Design review of the part built by this model. Coordinates are the model's own, in mm. Face numbers are marked on the shaded views. A direction names the side the tool comes from. Coordinates: 2 decimals unless noted, no trailing zeros. Loops run counter-clockwise (first coordinate to the right, second up) from the corner with the lowest first, then second, coordinate; pieces in that order, holes last. Notation, with made-up numbers: M 76,4 L 100,4 A8 cw 100,10 Z; hole C -10.75,37 d11. An arc over 180 degrees is marked long. Put each result on its own line as item: value. Start each with the question number.
(1) Take a section at B-B, the plane y = -11. Give the boundary of the cut face in (x, z).
(2) Clearance check with flat-ended pins moving along their axes: pin 1 (10 mm diameter, centred on x = -6, y = 5.5, fed in from -Z); pin 2 (2 mm diameter, centred on y = -0.5, z = -5.5, fed in from -X); pin 3 (2 mm diameter, centred on y = -11.5, z = -1.5, fed in from -X). State where each tip first meets the part, or that it passes through.
(3) Take a section at C-C, the plane z = -9.5. Give the boundary of the cut face in (x, y).
(4) Take a section at D-D, the plane y = 0. Give the boundary of the cut face in (x, z), then the cut area to 3 significant figures.
(5) The part is to be moulded in two halves that separate along Y. For the marked faces 3, 4 and 5, say which applies: +Y half, -Y half, draft (parallel to the pull), parting line (faces both ways), or undercut.
(6) Take a section at A-A, the plane x = 0. Give the boundary of the cut face in (y, z).
(7) For the marked faces 1 and 2, list the 3-axis set-ups (+Z, -Z, +X, -X, +Y, -Y) from which the entire face can be reached by the end or side of a thin tool; tool diameter is ignored.
(8) For probe 1 along Y at (x, z) = (0, 0.7); probe 2 along Y at (x, z) = (-12, -7.5); probe 3 along Z at (x, y) = (4, 8.5), list the stretches that pass through material, from the lowest coordinate up. Write a range as [from, to].
```python
from build123d import *

# Parameters (mm, degrees)
F0_W     = 40
F0_H     = 32
F0_R     = 6.25
F1_DEPTH = 2
F3_START = 13
F3_DEPTH = 3
F4_START = -13
F4_DEPTH = 3
F5_DEPTH = 16


with BuildPart() as f1:
    # F0 (on Top) → F1 (new body)
    with BuildSketch(Plane.XY):
        Rectangle(F0_W, F0_H)
        Circle(F0_R, mode=Mode.SUBTRACT)
    extrude(amount=F1_DEPTH)

    # F2 (on Front) → F3 (join)
    with BuildSketch(Plane.XZ.offset(F3_START)):
        with BuildLine():
            ThreePointArc((18.1261557407, -8.4523652348), (19.5259201424, -4.3287922788), (20, 0))
            Line((20, 0), (18.5, 0))
            ThreePointArc((18.5, 0), (18.0614761317, -4.0041328579), (16.7666940602, -7.8184378422))
            Line((16.7666940602, -7.8184378422), (18.1261557407, -8.4523652348))
        make_face()
        with BuildLine():
            Line((-18.5, 0), (-20, 0))
            ThreePointArc((-20, 0), (-19.5259201424, -4.3287922788), (-18.1261557407, -8.4523652348))
            Line((-18.1261557407, -8.4523652348), (-16.7666940602, -7.8184378422))
            ThreePointArc((-16.7666940602, -7.8184378422), (-18.0614761317, -4.0041328579), (-18.5, 0))
        make_face()
        with BuildLine():
            ThreePointArc((-18.1261557407, -8.4523652348), (0, -20), (18.1261557407, -8.4523652348))
            Line((18.1261557407, -8.4523652348), (16.7666940602, -7.8184378422))
            ThreePointArc((16.7666940602, -7.8184378422), (0, -18.5), (-16.7666940602, -7.8184378422))
            Line((-16.7666940602, -7.8184378422), (-18.1261557407, -8.4523652348))
        make_face()
        with BuildLine():
            ThreePointArc((16.7666940602, -7.8184378422), (18.0614761317, -4.0041328579), (18.5, 0))
            Line((18.5, 0), (0, 0))
            Line((0, 0), (16.7666940602, -7.8184378422))
        make_face()
        with BuildLine():
            Line((0, 0), (-18.5, 0))
            ThreePointArc((-18.5, 0), (-18.0614761317, -4.0041328579), (-16.7666940602, -7.8184378422))
            Line((-16.7666940602, -7.8184378422), (0, 0))
        make_face()
        with BuildLine():
            ThreePointArc((-16.7666940602, -7.8184378422), (0, -18.5), (16.7666940602, -7.8184378422))
            Line((16.7666940602, -7.8184378422), (0, 0))
            Line((0, 0), (-16.7666940602, -7.8184378422))
        make_face()
    extrude(amount=F3_DEPTH)

    # F2 (on Front) → F4 (join)
    with BuildSketch(Plane.XZ.offset(F4_START)):
        with BuildLine():
            ThreePointArc((18.1261557407, -8.4523652348), (19.5259201424, -4.3287922788), (20, 0))
            Line((20, 0), (18.5, 0))
            ThreePointArc((18.5, 0), (18.0614761317, -4.0041328579), (16.7666940602, -7.8184378422))
            Line((16.7666940602, -7.8184378422), (18.1261557407, -8.4523652348))
        make_face()
        with BuildLine():
            Line((-18.5, 0), (-20, 0))
            ThreePointArc((-20, 0), (-19.5259201424, -4.3287922788), (-18.1261557407, -8.4523652348))
            Line((-18.1261557407, -8.4523652348), (-16.7666940602, -7.8184378422))
            ThreePointArc((-16.7666940602, -7.8184378422), (-18.0614761317, -4.0041328579), (-18.5, 0))
        make_face()
        with BuildLine():
            ThreePointArc((-18.1261557407, -8.4523652348), (0, -20), (18.1261557407, -8.4523652348))
            Line((18.1261557407, -8.4523652348), (16.7666940602, -7.8184378422))
            ThreePointArc((16.7666940602, -7.8184378422), (0, -18.5), (-16.7666940602, -7.8184378422))
            Line((-16.7666940602, -7.8184378422), (-18.1261557407, -8.4523652348))
        make_face()
        with BuildLine():
            ThreePointArc((16.7666940602, -7.8184378422), (18.0614761317, -4.0041328579), (18.5, 0))
            Line((18.5, 0), (0, 0))
            Line((0, 0), (16.7666940602, -7.8184378422))
        make_face()
        with BuildLine():
            Line((0, 0), (-18.5, 0))
            ThreePointArc((-18.5, 0), (-18.0614761317, -4.0041328579), (-16.7666940602, -7.8184378422))
            Line((-16.7666940602, -7.8184378422), (0, 0))
        make_face()
        with BuildLine():
            ThreePointArc((-16.7666940602, -7.8184378422), (0, -18.5), (16.7666940602, -7.8184378422))
            Line((16.7666940602, -7.8184378422), (0, 0))
            Line((0, 0), (-16.7666940602, -7.8184378422))
        make_face()
    extrude(amount=-F4_DEPTH)

    # F2 (on Front) → F5 (join, symmetric)
    with BuildSketch(Plane.XZ):
        with BuildLine():
            ThreePointArc((18.1261557407, -8.4523652348), (19.5259201424, -4.3287922788), (20, 0))
            Line((20, 0), (18.5, 0))
            ThreePointArc((18.5, 0), (18.0614761317, -4.0041328579), (16.7666940602, -7.8184378422))
            Line((16.7666940602, -7.8184378422), (18.1261557407, -8.4523652348))
        make_face()
        with BuildLine():
            Line((-18.5, 0), (-20, 0))
            ThreePointArc((-20, 0), (-19.5259201424, -4.3287922788), (-18.1261557407, -8.4523652348))
            Line((-18.1261557407, -8.4523652348), (-16.7666940602, -7.8184378422))
            ThreePointArc((-16.7666940602, -7.8184378422), (-18.0614761317, -4.0041328579), (-18.5, 0))
        make_face()
    extrude(amount=F5_DEPTH, both=True)


solid = f1.part
```
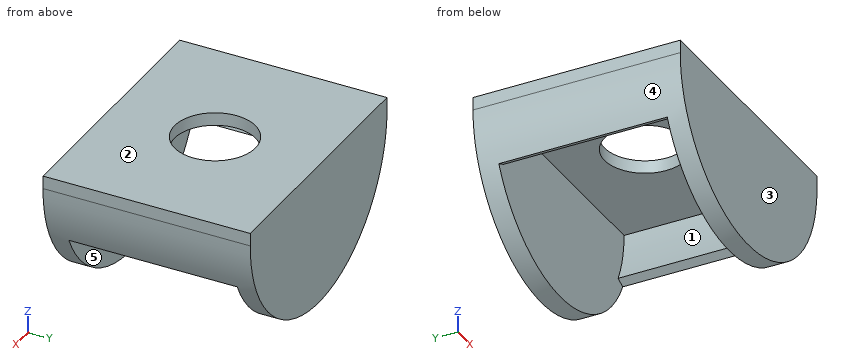
Computed values:
1. outline: M -20,0 A20 ccw -18.13,-8.45 L -16.77,-7.82 A18.5 cw -18.5,0 L 18.5,0 A18.5 cw 16.77,-7.82 L 18.13,-8.45 A20 ccw 20,0 L 20,2 L -20,2 Z
2. pin 1: stops at z = 0
2. pin 2: stops at x = -19.49
2. pin 3: stops at x = -19.99
3. outline: M -17.6,-16 L 17.6,-16 L 17.6,-13 L -17.6,-13 Z; M -17.6,13 L 17.6,13 L 17.6,16 L -17.6,16 Z
4. outline: M -20,0 A20 ccw -18.13,-8.45 L -16.77,-7.82 A18.5 cw -18.5,0 L -6.25,0 L -6.25,2 L -20,2 Z; M 6.25,0 L 18.5,0 A18.5 cw 16.77,-7.82 L 18.13,-8.45 A20 ccw 20,0 L 20,2 L 6.25,2 Z
4. area: 80.2 mm^2
5. face 3: -Y half
5. face 4: draft
5. face 5: undercut
6. outline: M -16,-20 L -13,-20 L -13,0 L -6.25,0 L -6.25,2 L -16,2 Z; M 6.25,0 L 13,0 L 13,-20 L 16,-20 L 16,2 L 6.25,2 Z
7. face 1: none
7. face 2: +Z, +X, -X, +Y, -Y
8. probe 1: y = [-16, -6.25], [6.25, 16]
8. probe 2: y = [-16, -13], [13, 16]
8. probe 3: z = [0, 2]
